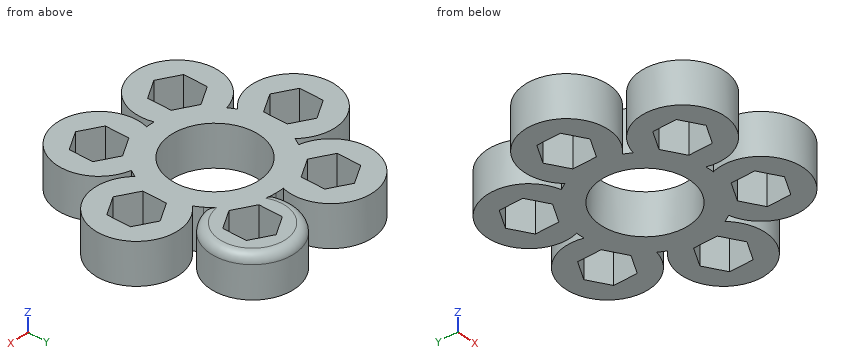
from build123d import *

# Parameters (mm, degrees)
F0_R        = 7.5
F1_DEPTH    = 7
F2_T4_ANGLE = 334.5116796515
F2_S5_R     = 10.95
F2_T6_DEPTH = 12


# Not quite as in the source:
# - a fillet or chamfer that OpenCascade refuses, or shapes differently, is made with other operations: its cross-section is extruded or revolved along the edge and cut away or added


with BuildPart() as f1:
    # F0 (on Top) → F1 (new body)
    with BuildSketch(Plane.XY):
        with BuildLine():
            ThreePointArc((-9.8156361058, 4.8534305226), (-22.1016488807, 0), (-9.8156361058, -4.8534305226))
            ThreePointArc((-9.8156361058, -4.8534305226), (-9.4829781714, -5.475), (-9.111012181, -6.0738749607))
            ThreePointArc((-9.111012181, -6.0738749607), (-11.0508244404, -19.1405893962), (-0.7046239248, -10.9273054833))
            ThreePointArc((-0.7046239248, -10.9273054833), (0, -10.95), (0.7046239248, -10.9273054833))
            ThreePointArc((0.7046239248, -10.9273054833), (11.0508244404, -19.1405893962), (9.111012181, -6.0738749607))
            ThreePointArc((9.111012181, -6.0738749607), (9.4829781714, -5.475), (9.8156361058, -4.8534305226))
            ThreePointArc((9.8156361058, -4.8534305226), (22.1016488807, 0), (9.8156361058, 4.8534305226))
            ThreePointArc((9.8156361058, 4.8534305226), (9.4829781714, 5.475), (9.111012181, 6.0738749607))
            ThreePointArc((9.111012181, 6.0738749607), (11.0508244404, 19.1405893962), (0.7046239248, 10.9273054833))
            ThreePointArc((0.7046239248, 10.9273054833), (0, 10.95), (-0.7046239248, 10.9273054833))
            ThreePointArc((-0.7046239248, 10.9273054833), (-11.0508244404, 19.1405893962), (-9.111012181, 6.0738749607))
            ThreePointArc((-9.111012181, 6.0738749607), (-9.4829781714, 5.475), (-9.8156361058, 4.8534305226))
        make_face()
        Polygon((-4.05, -14.9822394855), (-7.5, -16.9740979142), (-10.95, -14.9822394855), (-10.95, -10.9985226281), (-7.5, -9.0066641994), (-4.05, -10.9985226281), align=None, mode=Mode.SUBTRACT)
        Polygon((10.95, -10.9985226281), (10.95, -14.9822394855), (7.5, -16.9740979142), (4.05, -14.9822394855), (4.05, -10.9985226281), (7.5, -9.0066641994), align=None, mode=Mode.SUBTRACT)
        Polygon((-15, 3.9837168574), (-11.55, 1.9918584287), (-11.55, -1.9918584287), (-15, -3.9837168574), (-18.45, -1.9918584287), (-18.45, 1.9918584287), align=None, mode=Mode.SUBTRACT)
        Polygon((-10.95, 10.9985226281), (-10.95, 14.9822394855), (-7.5, 16.9740979142), (-4.05, 14.9822394855), (-4.05, 10.9985226281), (-7.5, 9.0066641994), align=None, mode=Mode.SUBTRACT)
        Circle(F0_R, mode=Mode.SUBTRACT)
        Polygon((15, 3.9837168574), (18.45, 1.9918584287), (18.45, -1.9918584287), (15, -3.9837168574), (11.55, -1.9918584287), (11.55, 1.9918584287), align=None, mode=Mode.SUBTRACT)
        Polygon((4.05, 14.9822394855), (7.5, 16.9740979142), (10.95, 14.9822394855), (10.95, 10.9985226281), (7.5, 9.0066641994), (4.05, 10.9985226281), align=None, mode=Mode.SUBTRACT)
    extrude(amount=F1_DEPTH)

    # F2: fillet of radius 1.5 on 1 edges, made by hand


with BuildPart() as f2_tool2:
    # F2_s3 → F2_t4 (revolve)
    with BuildSketch(Plane(origin=(3.1600326445, -0.9815693661, 0), x_dir=(0, 0, 1), z_dir=(-0.9549897147, 0.2966389131, 0))):
        with BuildLine():
            ThreePointArc((5.5, 7.528823267), (6.5606601718, 7.9681630952), (7, 9.028823267))
            Line((7, 9.028823267), (7, 7.528823267))
            Line((7, 7.528823267), (5.5, 7.528823267))
        make_face()
    revolve(axis=Axis((7.5, 12.9903810568, 7), (0, 0, 1)), revolution_arc=F2_T4_ANGLE)

    # F2_s5 → F2_t6 (cut, symmetric)
    with BuildSketch(Plane.XY.offset(6.2)):
        Circle(F2_S5_R)
    extrude(amount=F2_T6_DEPTH, both=True, mode=Mode.SUBTRACT)


with BuildPart() as f1_1:
    add(f1.part)

    # F2_t1: cut F2_tool2
    add(f2_tool2.part, mode=Mode.SUBTRACT)


solid = f1_1.part
Could you check a few things on this model? Use its own coordinates, in mm. Round coordinates to 2 decimals unless told otherwise and drop trailing zeros. Write each loop counter-clockwise with the first axis right and the second up, starting at its lowest first coordinate (ties: lowest second). Pieces come first, ordered by that corner, then holes. Notation, with made-up numbers: (14.25, -30) - (66.25, -30) arc R13 cw to (66.25, -6) - close; hole circle Ø3 at (7, 78.25). An arc over 180 degrees is marked (long way). Put each result on its own line as item: value. Start each with the question number.
(1) I want a section at A-A, the plane y = 0. Please give me the cut outline in (x, z).
(2) I need wall thicknesses on probe 1 along Y at (x, z) = (0, 1.75); probe 2 along X at (y, z) = (-16, 1.75); probe 3 along Y at (x, z) = (13, 5). Which ranges of each line are inside material? Lowest first, please.
(3) I want a section at B-B, the plane x = -3.5. Please give me the cut outline in (y, z).
(4) I want a section at C-C, the plane z = 2.75. Give the number of separate pieces and of enclosed holes in the cut face, plus the area to 3 significant figures.
(5) Will these pins go through, and if not, where does the flat tip stop? pin 1 (2 mm diameter, centred on y = -14, z = 2.5, fed in from +X); pin 2 (4 mm diameter, centred on y = -6.5, z = 6, fed in from -X); pin 3 (2 mm diameter, centred on x = 10.5, z = 4, fed in from +Y); pin 4 (12 mm diameter, centred on x = 0, y = 0, fed in from +Z).
Here are the results:
1. outline: (-22.1, 0) - (-18.45, 0) - (-18.45, 7) - (-22.1, 7) - close; (-11.55, 0) - (-7.5, 0) - (-7.5, 7) - (-11.55, 7) - close; (7.5, 0) - (11.55, 0) - (11.55, 7) - (7.5, 7) - close; (18.45, 0) - (22.1, 0) - (22.1, 7) - (18.45, 7) - close
2. probe 1: y = -10.95 to -7.5, 7.5 to 10.95
2. probe 2: x = -13.93 to -9.19, -5.81 to -1.07, 1.07 to 5.81, 9.19 to 13.93
2. probe 3: y = -17.48 to -8.5, -6.81 to -2.83, 2.83 to 6.81, 8.5 to 17.48
3. outline: (-18.86, 0) - (-6.63, 0) - (-6.63, 7) - (-18.86, 7) - close; (6.63, 0) - (18.86, 0) - (18.86, 7) - (6.63, 7) - close
4. separate pieces: 1
4. enclosed holes: 7
4. area: 782 mm^2
5. pin 1: stops at x = 14.6
5. pin 2: stops at x = -20.49
5. pin 3: stops at y = 19.8
5. pin 4: passes through
